```python
from build123d import *

# Parameters (mm, degrees)
SKETCH6_R               = 6
BOSS_EXTRUDE4_DEPTH     = 2.5
SKETCH7_R               = 6.1
BOSS_EXTRUDE5_DEPTH     = 5.2
SKETCH8_R               = 6.05
BOSS_EXTRUDE6_DEPTH     = 5.2
SKETCH13_R              = 10
BOSS_EXTRUDE7_DEPTH     = 5
CUT_EXTRUDE1_DEPTH      = 6.2
CUT_EXTRUDE1_DEPTH_BACK = 11.2
CHAMFER1_SIZE           = 0.5


with BuildPart() as part:
    # Sketch6 → Boss-Extrude4 (new body, symmetric)
    with BuildSketch(Plane.XY):
        Circle(SKETCH6_R)
    extrude(amount=BOSS_EXTRUDE4_DEPTH, both=True)

    # Sketch7 → Boss-Extrude5 (add)
    with BuildSketch(Plane.XY.offset(2.5)):
        with Locations((0, 1)):
            Circle(SKETCH7_R)
    extrude(amount=BOSS_EXTRUDE5_DEPTH)

    # Sketch8 → Boss-Extrude6 (add)
    with BuildSketch(Plane(origin=(0, 0, -2.5), x_dir=(-1, 0, 0), z_dir=(0, 0, -1))):
        with Locations((0, -1)):
            Circle(SKETCH8_R)
    extrude(amount=BOSS_EXTRUDE6_DEPTH)

    # Sketch13 → Boss-Extrude7 (add)
    with BuildSketch(Plane.XY.offset(2.5)):
        Circle(SKETCH13_R)
    extrude(amount=-BOSS_EXTRUDE7_DEPTH)

    # Sketch11 → Cut-Extrude1 (cut, two sides)
    with BuildSketch(Plane.XY.offset(2.5)) as cut_extrude1_sk:
        with BuildLine():
            Line((-2.886607005, -1.7), (2.886607005, -1.7))
            ThreePointArc((2.886607005, -1.7), (3.35, 0), (2.886607005, 1.7))
            Line((2.886607005, 1.7), (-2.886607005, 1.7))
            ThreePointArc((-2.886607005, 1.7), (-3.35, 0), (-2.886607005, -1.7))
        make_face()
    extrude(amount=CUT_EXTRUDE1_DEPTH, mode=Mode.SUBTRACT)
    extrude(cut_extrude1_sk.sketch, amount=-CUT_EXTRUDE1_DEPTH_BACK, mode=Mode.SUBTRACT)

    # Chamfer1
    chamfer1_edges = [part.edges().sort_by_distance(p)[0] for p in [
        (6.05, -1, -7.7),
        (-6.1, 1, 7.7),
    ]]
    chamfer(chamfer1_edges, length=CHAMFER1_SIZE)


solid = part.part
```
Source: CAD feature listing. Evaluate the final solid. Frame: model axes, mm. A direction names the side the tool comes from. Give positions to 0.01 mm unless a question says otherwise; leave off trailing zeros. Loops run counter-clockwise (first coordinate to the right, second up) from the corner with the lowest first, then second, coordinate; pieces in that order, holes last. Notation, with made-up numbers: (83, 6) -> (132, 6) arc R24 ccw to (132, 32) -> close; hole circle Ø10 at (59, 44.5). An arc over 180 degrees is marked (long way). Put each result on its own line as item: value. Start each with the question number.
1) Cut plane D-D (y = -8.25). Return loops of the section in (x, z), then the cut area to 3 significant figures.
2) Contact query for flat-ended pins moving along their axis: P1, Ø3, axis at y = -6, z = 0, coming from the -X side; P2, Ø2, axis at y = 7, z = -4, coming from the -X side; P3, Ø1.5, axis at y = 5, z = 5.5, coming from the +X side; P4, Ø1, axis at y = -4, z = 4, coming from the -X side. Output: stop coordinate, or through.
3) Reachability of faces 4 (the face through (-2, 5, -2.5)), 5 (the face through (0, 2, 7.7)), 6 (the face through (0, 1.7, 0)), 7 (the face through (3.279, 6.144, 4.817)) from +Z, -Z, +X, -X, +Y, -Y: full face, straight path, thin tool, end or side. Return the list, or none.
4) Cut plane C-C (z = 4.5). Return loops of the section in (x, y).
5) Material intervals for probe 1 along Y at (x, z) = (0, -3); probe 2 along Z at (x, y) = (-8.5, 4.75); probe 3 along Y at (x, z) = (3, 5), sorted ascending.
6) Draft query along X for faces 1 (the face through (-3.35, 0.02, -0.11)), 2 (the face through (0, -2, -7.7)), 3 (the face through (-5.77, 0.82, -4.82)). Return one class per face: released by +X, released by -X, zero draft, split by the parting line, or undercut.
7) Cut plane B-B (z = -4). Return loops of the section in (x, y), then the cut area to 3 significant figures.
8) Cut plane A-A (x = 0). Return loops of the section in (y, z).
Results are:
1. outline: (-5.65, -2.5) -> (5.65, -2.5) -> (5.65, 2.5) -> (-5.65, 2.5) -> close
1. area: 56.5 mm2
2. P1: stops at x = -8.93
2. P2: passes through
2. P3: stops at x = 5.16
2. P4: stops at x = -4.12
3. face 4: -Z
3. face 5: +Z, +X, -X, +Y, -Y
3. face 6: +Z, -Z
3. face 7: +Z
4. outline: circle Ø12.2 at (0, 1); hole (-2.89, -1.7) -> (2.89, -1.7) arc R3.35 ccw to (2.89, 1.7) -> (-2.89, 1.7) arc R3.35 ccw to start
5. probe 1: y = -7.05 to -1.7, 1.7 to 5.05
5. probe 2: z = -2.5 to 2.5
5. probe 3: y = -4.31 to -1.49, 1.49 to 6.31
6. face 1: undercut
6. face 2: zero draft
6. face 3: split by the parting line
7. outline: circle Ø12.1 at (0, -1); hole (-2.89, -1.7) -> (2.89, -1.7) arc R3.35 ccw to (2.89, 1.7) -> (-2.89, 1.7) arc R3.35 ccw to start
7. area: 93.2 mm2
8. outline: (-10, -2.5) -> (-7.05, -2.5) -> (-7.05, -7.2) -> (-6.55, -7.7) -> (-1.7, -7.7) -> (-1.7, 7.7) -> (-4.6, 7.7) -> (-5.1, 7.2) -> (-5.1, 2.5) -> (-10, 2.5) -> close; (1.7, -7.7) -> (4.55, -7.7) -> (5.05, -7.2) -> (5.05, -2.5) -> (10, -2.5) -> (10, 2.5) -> (7.1, 2.5) -> (7.1, 7.2) -> (6.6, 7.7) -> (1.7, 7.7) -> close
